Here's how the part is built. I have some questions about the finished solid (model axes, mm). A direction names the side the tool comes from. Coordinates: 2 decimals unless noted, no trailing zeros. Write each loop counter-clockwise with the first axis right and the second up, starting at its lowest first coordinate (ties: lowest second). Pieces come first, ordered by that corner, then holes.
(1) Imagine slicing it at A-A, the plane z = 0. List the corners of the cut face in (x, y) for me.
(2) Imagine slicing it at D-D, the plane x = 35. List the corners of the cut face in (y, z) for me, plus the area to 3 significant figures.
(3) Thinking about a two-plate mould opening in Z: for faces 1 (the cylindrical face through (-0.1, 4.9, 63.5)), 2 (the flat face through (2.95, 4.93, 33.71)), 3 (the flat face through (-4, 10, 2)), 4 (the cylindrical face through (55.031, 4.93, -31.683)), which applies, released by +Z, released by -Z, zero draft, split by the parting line, or undercut?
(4) For pin 1 Ø2 at (y, z) = (4.5, -0.5) entering from +X; pin 2 Ø4 at (x, y) = (41, 3) entering from -Z; pin 3 Ø4 at (x, y) = (3.5, 1) entering from -Z, each with a flat end and sliding along its axis, tell me the tip position at first contact or that it passes through.
(5) Please list where these lines run through material, in increasing order: probe 1 along X at (y, z) = (5, 0); probe 2 along X at (y, z) = (4.75, -2); probe 3 along Z at (x, y) = (-12, 9).
(6) Imagine slicing it at B-B, the plane y = 4.5. List the corners of the cut face in (x, z) for me, plus the area to 3 significant figures.
(7) Imagine slicing it at C-C, the plane z = 56.5. List the corners of the cut face in (x, y) for me, plus the area to 3 significant figures.
(8) Which directions (+Z, -Z, +X, -X, +Y, -Y) give clear straight access to the entire face, cutting with the end or side of a thin tool? Please do faces 5 (the flat face through (-3.02, 4.93, 34.53)), 6 (the flat face through (27.72, 4.93, -19.41)), 7 (the flat face through (-4, 0, 2)).
```python
from build123d import *

# Parameters (mm, degrees)
SKETCH1_R           = 63.5
SKETCH1_R_2         = 2.6
BOSS_EXTRUDE1_DEPTH = 10
CUT_EXTRUDE1_START  = -10
CUT_EXTRUDE1_DEPTH  = 10


with BuildPart() as part:
    # Sketch1 → Boss-Extrude1 (new body)
    with BuildSketch(Plane(origin=(0, 0, 0), x_dir=(1, 0, 0), z_dir=(0, 1, 0))):
        with Locations(Location((0, 0, 0), (0, 0, 270))):
            Circle(SKETCH1_R)
        with Locations(Location((0, 0, 0), (0, 0, 270))):
            Circle(SKETCH1_R_2, mode=Mode.SUBTRACT)
    extrude(amount=BOSS_EXTRUDE1_DEPTH)

    # Sketch2 → Cut-Extrude1 (cut)
    with BuildSketch(Plane(origin=(0, 10, 0), x_dir=(1, 0, 0), z_dir=(0, 1, 0)).offset(CUT_EXTRUDE1_START)):
        with BuildLine():
            ThreePointArc((4.531538935, 2.113091309), (4.330127019, -2.5), (0.435778714, -4.98097349))
            Line((0.435778714, -4.98097349), (5.534389664, -63.258363329))
            ThreePointArc((5.534389664, -63.258363329), (54.99261314, -31.75), (57.550544477, 26.836259621))
            Line((57.550544477, 26.836259621), (4.531538935, 2.113091309))
        make_face()
        with BuildLine():
            Line((-5.534389664, -63.258363329), (-0.435778714, -4.98097349))
            ThreePointArc((-0.435778714, -4.98097349), (-4.330127019, -2.5), (-4.531538935, 2.113091309))
            Line((-4.531538935, 2.113091309), (-57.550544477, 26.836259621))
            ThreePointArc((-57.550544477, 26.836259621), (-54.99261314, -31.75), (-5.534389664, -63.258363329))
        make_face()
        with BuildLine():
            Line((-52.016154812, 36.422103708), (-4.095760221, 2.867882182))
            ThreePointArc((-4.095760221, 2.867882182), (0, 5), (4.095760221, 2.867882182))
            Line((4.095760221, 2.867882182), (52.016154812, 36.422103708))
            ThreePointArc((52.016154812, 36.422103708), (0, 63.5), (-52.016154812, 36.422103708))
        make_face()
    extrude(amount=CUT_EXTRUDE1_DEPTH, mode=Mode.SUBTRACT)


solid = part.part
```
Recorded:
1. outline: (-5, 0) - (-2.6, 0) - (-2.6, 10) - (-5, 10) - close; (2.6, 0) - (5, 0) - (5, 10) - (2.6, 10) - close
2. outline: (0, -24.51) - (10, -24.51) - (10, -16.32) - (0, -16.32) - close
2. area: 81.9 mm2
3. face 1: released by +Z
3. face 2: undercut
3. face 3: zero draft
3. face 4: released by -Z
4. pin 1: stops at x = 5
4. pin 2: stops at z = -30.11
4. pin 3: stops at z = -4.77
5. probe 1: x = -5 to -2.6, 2.6 to 5
5. probe 2: x = -4.58 to -1.66, 1.66 to 4.58
5. probe 3: z = -8.4 to -5.6
6. outline: (-57.55, -26.84) arc R63.5 ccw to (-52.02, -36.42) - (-4.1, -2.87) arc R5 ccw to (4.1, -2.87) - (52.02, -36.42) arc R63.5 ccw to (57.55, -26.84) - (4.53, -2.11) arc R5 ccw to (0.44, 4.98) - (5.53, 63.26) arc R63.5 ccw to (-5.53, 63.26) - (-0.44, 4.98) arc R5 ccw to (-4.53, -2.11) - close; hole circle Ø5.2 at (0, 0)
6. area: 1,110 mm2
7. outline: (-4.94, 0) - (4.94, 0) - (4.94, 10) - (-4.94, 10) - close
7. area: 98.9 mm2
8. face 5: -X, +Y, -Y
8. face 6: -Z, +Y, -Y
8. face 7: +Z, -Z, +X, -X, -Y
